Can you work these out from the model? Positions are in its coordinate system, mm. A direction names the side the tool comes from. Give positions to 0.01 mm unless a question says otherwise; leave off trailing zeros. Write each loop counter-clockwise with the first axis right and the second up, starting at its lowest first coordinate (ties: lowest second). Pieces come first, ordered by that corner, then holes.
1. I'm going to push flat-ended pins straight in: pin 1 (8 mm diameter, centred on x = -7.5, y = 25, fed in from -Z); pin 2 (2 mm diameter, centred on y = 22.5, z = 6.5, fed in from -X); pin 3 (1 mm diameter, centred on x = 11, y = 11.5, fed in from +Z). Where does each tip first touch, or does it pass through?
2. On a 3-axis mill with a long thin cutter (end or side, diameter ignored), from which of +Z, -Z, +X, -X, +Y, -Y can I reach the whole of each face in a straight line? I mean faces 1 (the flat face through (-10, 0, 13)), 2 (the cylindrical face through (-14.004, 50.441, 23.379)). Say none if no direction works.
3. Suppose I cut it at A-A (x = 0). Please give me the cut outline in (y, z).
4. Suppose I cut it at D-D (x = 4). Please give me the cut outline in (y, z), and give its area (3 significant figures).
5. Thinking about a two-plate mould opening in Z: for faces 3 (the flat face through (-9, 24, 38.7)), 4 (the cylindrical face through (-2.47, 37.07, -18.84)), 5 (the cylindrical face through (-2.083, 37.074, -15.864)), which applies, pulls with the +Z half, pulls with the -Z half, needs draft (parallel to the pull), parting line crosses it, or undercut?
6. Suppose I cut it at B-B (z = -3.5). Please give me the cut outline in (x, y), and give its area (3 significant figures).
7. If I drill on probe 1 along Y at (x, z) = (0, 30.5); probe 2 along X at (y, z) = (60, 0); probe 3 along Z at (x, y) = (-0.5, 68.5), over which ranges is the centre line in solid material (lowest first)?
8. Suppose I cut it at C-C (y = 37.6). Please give me the cut outline in (x, z), and give its area (3 significant figures).
```python
from build123d import *

# Parameters (mm, degrees)
SKETCH_1_R          = 19
SKETCH_1_R_2        = 16
EXTRUDE_1_DEPTH     = 75.2
SKETCH_2_R          = 19
SKETCH_2_R_2        = 16
EXTRUDE_2_DEPTH     = 38.7
SKETCH_3_R          = 16
CUT_EXTRUDE_1_DEPTH = 76.2000001
CUT_EXTRUDE_2_REACH = 59.7
SKETCH_4_R          = 16


with BuildPart() as part:
    # 草图1 → 凸台-拉伸1 (new body)
    with BuildSketch(Plane(origin=(0, 0, 0), x_dir=(1, 0, 0), z_dir=(0, 1, 0))):
        Circle(SKETCH_1_R)
        Circle(SKETCH_1_R_2, mode=Mode.SUBTRACT)
    extrude(amount=EXTRUDE_1_DEPTH)

    # 草图2 → 凸台-拉伸2 (add)
    with BuildSketch(Plane.XY):
        with Locations((0, 37.6)):
            Circle(SKETCH_2_R)
        with Locations((0, 37.6)):
            Circle(SKETCH_2_R_2, mode=Mode.SUBTRACT)
    extrude(amount=EXTRUDE_2_DEPTH)

    # 草图3 → 切除-拉伸1 (cut, through all)
    with BuildSketch(Plane(origin=(0, 75.2, 0), x_dir=(1, 0, 0), z_dir=(0, 1, 0))):
        Circle(SKETCH_3_R)
    extrude(amount=-CUT_EXTRUDE_1_DEPTH, mode=Mode.SUBTRACT)

    # 草图4 → 切除-拉伸2 (cut, up to next)
    with BuildSketch(Plane.XY.offset(38.7), mode=Mode.PRIVATE) as cut_extrude_2_sk1:
        with Locations((0, 37.6)):
            Circle(SKETCH_4_R)
    cut_extrude_2_tool1 = extrude(cut_extrude_2_sk1.sketch, amount=-CUT_EXTRUDE_2_REACH, mode=Mode.PRIVATE) & part.part
    add(cut_extrude_2_tool1.solids().sort_by_distance((0, 37.6, 38.7))[0], mode=Mode.SUBTRACT)


solid = part.part
```
Checks:
1. pin 1: stops at z = -18.67
1. pin 2: stops at x = -18.19
1. pin 3: stops at z = 15.84
2. face 1: +Z, -Z, +X, -X, -Y
2. face 2: +Z
3. outline: (0, -19) - (75.2, -19) - (75.2, -16) - (0, -16) - close; (0, 16) - (21.6, 16) - (21.6, 38.7) - (18.6, 38.7) - (18.6, 19) - (0, 19) - close; (53.6, 16) - (75.2, 16) - (75.2, 19) - (56.6, 19) - (56.6, 38.7) - (53.6, 38.7) - close
4. outline: (0, -18.57) - (75.2, -18.57) - (75.2, -15.49) - (0, -15.49) - close; (0, 15.49) - (22.11, 15.49) - (22.11, 38.7) - (19.03, 38.7) - (19.03, 18.57) - (0, 18.57) - close; (53.09, 15.49) - (75.2, 15.49) - (75.2, 18.57) - (56.17, 18.57) - (56.17, 38.7) - (53.09, 38.7) - close
4. area: 492 mm2
5. face 3: pulls with the +Z half
5. face 4: parting line crosses it
5. face 5: undercut
6. outline: (-18.67, 0) - (-15.61, 0) - (-15.61, 75.2) - (-18.67, 75.2) - close; (15.61, 0) - (18.67, 0) - (18.67, 75.2) - (15.61, 75.2) - close
6. area: 461 mm2
7. probe 1: y = 18.6 to 21.6, 53.6 to 56.6
7. probe 2: x = -19 to -16, 16 to 19
7. probe 3: z = -18.99 to -15.99, 15.99 to 18.99
8. outline: (-19, 0) arc R19 ccw to (19, 0) - (19, 38.7) - (16, 38.7) - (16, 0) arc R16 cw to (-16, 0) - (-16, 38.7) - (-19, 38.7) - close
8. area: 397 mm2
